from build123d import *

# Parameters (mm, degrees)
F0_R     = 11.25
F1_DEPTH = 7
F2_R     = 2.5


with BuildPart() as f1:
    # F0 (on Top) → F1 (new body)
    with BuildSketch(Plane.XY):
        with BuildLine():
            ThreePointArc((8.929492, -12.589746), (11.341301, -11.590742), (13.929492, -11.25))
            Line((13.929492, -11.25), (30, -11.25))
            ThreePointArc((30, -11.25), (37.071068, -8.321068), (40, -1.25))
            Line((40, -1.25), (40, 1.25))
            ThreePointArc((40, 1.25), (37.071068, 8.321068), (30, 11.25))
            Line((30, 11.25), (13.929492, 11.25))
            ThreePointArc((13.929492, 11.25), (11.341301, 11.590742), (8.929492, 12.589746))
            Line((8.929492, 12.589746), (6.438294, 14.02804))
            ThreePointArc((6.438294, 14.02804), (4.367226, 15.617226), (2.77804, 17.688294))
            Line((2.77804, 17.688294), (-5.257214, 31.605762))
            ThreePointArc((-5.257214, 31.605762), (-11.329278, 36.26502), (-18.917468, 35.266016))
            Line((-18.917468, 35.266016), (-21.082532, 34.016016))
            ThreePointArc((-21.082532, 34.016016), (-25.74179, 27.943953), (-24.742786, 20.355762))
            Line((-24.742786, 20.355762), (-16.707532, 6.438294))
            ThreePointArc((-16.707532, 6.438294), (-15.708528, 4.026484), (-15.367786, 1.438294))
            Line((-15.367786, 1.438294), (-15.367786, -1.438294))
            ThreePointArc((-15.367786, -1.438294), (-15.708528, -4.026484), (-16.707532, -6.438294))
            Line((-16.707532, -6.438294), (-24.742786, -20.355762))
            ThreePointArc((-24.742786, -20.355762), (-25.74179, -27.943953), (-21.082532, -34.016016))
            Line((-21.082532, -34.016016), (-18.917468, -35.266016))
            ThreePointArc((-18.917468, -35.266016), (-11.329278, -36.26502), (-5.257214, -31.605762))
            Line((-5.257214, -31.605762), (2.77804, -17.688294))
            ThreePointArc((2.77804, -17.688294), (4.367226, -15.617226), (6.438294, -14.02804))
            Line((6.438294, -14.02804), (8.929492, -12.589746))
        make_face()
        Circle(F0_R, mode=Mode.SUBTRACT)
    extrude(amount=F1_DEPTH)

    # F2
    f2_edges = [f1.edges().sort_by_distance(p)[0] for p in [
        (-1.239587, -24.647028, 7),
        (21.964746, 11.25, 0),
    ]]
    fillet(f2_edges, radius=F2_R)


solid = f1.part
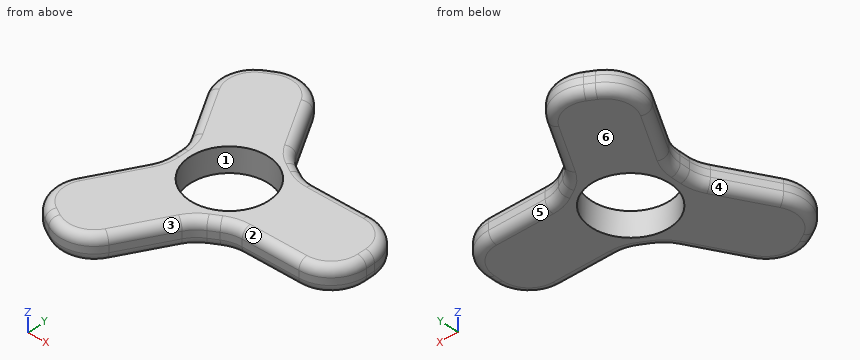
Verification items for the finished model (mm, model axes). Face numbers are marked on the shaded views. A direction names the side the tool comes from. Round coordinates to 2 decimals unless told otherwise and drop trailing zeros. Loops run counter-clockwise (first coordinate to the right, second up) from the corner with the lowest first, then second, coordinate; pieces in that order, holes last. Notation, with made-up numbers: (-10.75, 83.5) - (19.25, 83.5) arc R35 ccw to (19.25, 121.5) - close; hole circle Ø6 at (55, -16). An arc over 180 degrees is marked (long way). Use one line per item in the form item = value.
1. Scan lines: probe 1 along Y at (x, z) = (-9, 1.5); probe 2 along Y at (x, z) = (0, 4); probe 3 along X at (y, z) = (-5, 5.25). Record each from-to range of solid material in increasing order.
A:
probe_1 = -35.07 to -6.75, 6.75 to 35.07
probe_2 = -22.5 to -11.25, 11.25 to 22.5
probe_3 = -15.9 to -10.08, 10.08 to 39.15
2. Section check B-B on z = 3.5. Record the cut outline in (x, y).
A:
outline = (-24.74, -20.36) arc R10 ccw to (-21.08, -34.02) - (-18.92, -35.27) arc R10 ccw to (-5.26, -31.61) - (2.78, -17.69) arc R10 cw to (6.44, -14.03) - (8.93, -12.59) arc R10 cw to (13.93, -11.25) - (30, -11.25) arc R10 ccw to (40, -1.25) - (40, 1.25) arc R10 ccw to (30, 11.25) - (13.93, 11.25) arc R10 cw to (8.93, 12.59) - (6.44, 14.03) arc R10 cw to (2.78, 17.69) - (-5.26, 31.61) arc R10 ccw to (-18.92, 35.27) - (-21.08, 34.02) arc R10 ccw to (-24.74, 20.36) - (-16.71, 6.44) arc R10 cw to (-15.37, 1.44) - (-15.37, -1.44) arc R10 cw to (-16.71, -6.44) - close; hole circle Ø22.5 at (0, 0)
3. Section check A-A on y = 0. Record the cut outline in (x, z), and give its area (3 significant figures).
A:
outline = (-15.37, 2.5) arc R2.5 ccw to (-12.87, 0) - (-11.25, 0) - (-11.25, 7) - (-12.87, 7) arc R2.5 ccw to (-15.37, 4.5) - close; (11.25, 0) - (37.5, 0) arc R2.5 ccw to (40, 2.5) - (40, 4.5) arc R2.5 ccw to (37.5, 7) - (11.25, 7) - close
area = 225 mm²
4. Gauge pin test, flat ends, axial feed: pin 1 Ø4 at (x, z) = (14, 1) entering from -Y; pin 2 Ø1.5 at (y, z) = (-24, 6) entering from -X; pin 3 Ø1 at (y, z) = (0, 4) entering from -X; pin 4 Ø2 at (x, y) = (11, 0) entering from -Z. Record the tip position at first contact, or that the pin passes through.
A:
pin_1 = -11.35
pin_2 = -25.89
pin_3 = -15.37
pin_4 = 0
5. Section check C-C on x = 28. Record the cut outline in (y, z).
A:
outline = (-11.25, 2.5) arc R2.5 ccw to (-8.75, 0) - (8.75, 0) arc R2.5 ccw to (11.25, 2.5) - (11.25, 4.5) arc R2.5 ccw to (8.75, 7) - (-8.75, 7) arc R2.5 ccw to (-11.25, 4.5) - close
6. Access from +Z, -Z, +X, -X, +Y, -Y to the whole of each face (thin tool, end or side, straight path). Record for the marked faces 4, 5 and 6.
A:
face_4 = -Z, -X
face_5 = -Z, +X, +Y
face_6 = -Z, +X, -X, +Y, -Y
7. Draft check along X on the marked faces 1, 2 and 3. Enter one of: pulls with the +X half, pulls with the -X half, needs draft (parallel to the pull), parting line crosses it, or undercut.
A:
face_1 = undercut
face_2 = needs draft
face_3 = pulls with the +X half
